The listing builds one solid part. Answer for the finished solid, in the listing's coordinates (mm). A direction names the side the tool comes from. Give positions to 0.01 mm unless a question says otherwise; leave off trailing zeros. Order: outer loops, then holes, each group sorted by start corner. A loop starts at its lowest first (then second) coordinate and runs counter-clockwise, first axis right, second up. Notation, with made-up numbers: (-31, -22) - (12, -22) arc R8 ccw to (12, -17) - close; hole circle Ø11 at (80, -27). An arc over 180 degrees is marked (long way). Answer as a JSON object with one key per item and string values. Group by question number.
Q1. Given pin 1 (12 mm diameter, centred on x = -0.5, y = 24.5, fed in from +Z); pin 2 (1 mm diameter, centred on x = 4.5, z = 24, fed in from +Y); pin 3 (4.5 mm diameter, centred on y = 32.5, z = 0, fed in from -X), each flat-ended and moving along its own axis, determine where each tip first touches the part or whether it passes through.
Q2. The mould has two halves that part along X. Classify faces 1 (the face through (-24, 0, 0)), 2 (the face through (0.215, 34.136, -18.768)), 3 (the face through (-20, 31, -1)): released by +X, released by -X, zero draft, split by the parting line, or undercut.
Q3. A cutting plane is placed at B-B, the plane y = 3. Give the vertices of the cut face in (x, z).
Q4. Consider line 1 (X direction, y = 34, z = 7); line 2 (X direction, y = 3.5, z = 17); line 3 (Z direction, x = 8, y = 8). Determine where each line is inside the solid, lowest interval first.
Q5. A cutting plane is placed at A-A, the plane z = 0. Count the separate pieces of the cut face and the enclosed holes in it, and give its area (3 significant figures).
Q6. For faces 4 (the face through (22.5, 9, 0)), 5 (the face through (0, 0, -24)), 6 (the face through (-0.2, 34.3, 17.5)), 7 (the face through (0, 18, 23)), determine the directions among +Z, -Z, +X, -X, +Y, -Y from which every point of the face is accessible in a straight line to the end or side of a thin tool.
Autodesk Inventor part; units mm, degrees
ref_plane "Work Plane1" through (0, 17.75, 0) normal (0, 1, 0) x (1, 0, 0)
ref_plane "YZ Plane" through (0, 0, 0) normal (1, 0, 0) x (0, 1, 0)
ref_plane "XZ Plane" through (0, 0, 0) normal (0, 1, 0) x (-1, 0, 0)
sketch "Sketch1" plane through (0, 0, 0) normal (0, 1, 0) x (-1, 0, 0)
  line L0 (25, 25) -> (-25, 25)
  line L1 (-25, 25) -> (-25, -25)
  line L2 (-25, -25) -> (25, -25)
  line L3 (25, -25) -> (25, 25)
  line L4 (25, 25) -> (-25, -25) construction
  line L5 (-25, 25) -> (25, -25) construction
  line L6 (-22.5, 22.5) -> (22.5, 22.5)
  line L7 (22.5, 22.5) -> (22.5, -22.5)
  line L8 (22.5, -22.5) -> (-22.5, -22.5)
  line L9 (-22.5, -22.5) -> (-22.5, 22.5)
  line L10 (-22.5, 22.5) -> (22.5, -22.5) construction
  line L11 (22.5, 22.5) -> (-22.5, -22.5) construction
  point P0 (0, 0)
  dimension "d0" = 50
  dimension "d1" = 50
  dimension "d2" = 45
  dimension "d3" = 45
extrude "Extrusion1" add sketch "Sketch1" along normal blind 30
extrude "Extrusion2" add sketch "Sketch1" along normal blind 2 contours L6 L7 L8 L9
sketch "Sketch2" plane through (0, 30, 0) normal (0, 1, 0) x (1, 0, 0)
  point P0 (0, 0)
sketch "Sketch3" plane through (0, 30, 0) normal (0, 1, 0) x (1, 0, 0)
  line L0 (17.5, -17.5) -> (-17.5, -17.5)
  line L1 (-17.5, -17.5) -> (-17.5, 17.5)
  line L2 (-17.5, 17.5) -> (17.5, 17.5)
  line L3 (17.5, 17.5) -> (17.5, -17.5)
  line L4 (17.5, -17.5) -> (-17.5, 17.5) construction
  line L5 (-17.5, -17.5) -> (17.5, 17.5) construction
  line L6 (-25, 25) -> (-25, -25)
  line L7 (25, -25) -> (-25, -25)
  line L8 (-25, -25) -> (-25, 25)
  line L9 (-25, 25) -> (25, 25)
  line L10 (25, 25) -> (25, -25)
  line L11 (25, -25) -> (-25, 25) construction
  line L12 (-25, -25) -> (25, 25) construction
  point P0 (0, 0)
  dimension "d8" = 35
  dimension "d9" = 35
extrude "Extrusion3" add sketch "Sketch3" along normal blind 5.5
ref_plane "Work Plane1" through (0, 17.75, 0) normal (0, 1, 0) x (1, 0, 0)
chamfer "Chamfer1" distance 5 distance2 13.25 4 edges at (22.5, 30, 0) (0, 30, -22.5) (-22.5, 30, 0) (0, 30, 22.5) measured on face at (-5.8333, 30, 20.8333)
sketch "Sketch5" plane through (0, 35.5, 0) normal (0, 1, 0) x (1, 0, 0)
  point P0 (0, 0)
sketch "Sketch6" plane through (-17.5, 35.5, -17.5) normal (0, 0, 1) x (1, 0, 0)
  circle A0 centre (17.5, -3) radius 1.5
  line L0 (0, 0) -> (35, 0)
  point P0 (17.5, -35.5)
  point P1 (17.5, 0)
  dimension "d21" = 3
  dimension "d30" = 3
extrude "Extrusion5" cut sketch "Sketch6" against normal through all
sketch "Sketch7" plane through (0, 35.5, 0) normal (0, 1, 0) x (1, 0, 0)
  line L0 (25, 25) -> (-25, 25)
  line L1 (10, 25) -> (0, 25)
  line L2 (10, 25) -> (-10, 25)
  line L3 (-10, 25) -> (10, 25)
  line L4 (10, 25) -> (10, 23)
  line L5 (10, 23) -> (-10, 23)
  line L6 (-10, 23) -> (-10, 25)
  point P0 (0, 0)
  dimension "d24" = 20
  dimension "d25" = 2
extrude "Extrusion6" cut sketch "Sketch7" against normal through all
sketch "Sketch9" plane through (10, 35.5, -23) normal (0, 0, -1) x (-1, 0, 0)
  circle A0 centre (10, -3) radius 1.5
  circle A1 centre (10, -3) radius 2.5
  point P0 (10, -35.5)
  dimension "d37" = 3
extrude "Extrusion7" cut sketch "Sketch9" against normal blind 3
pattern_circular "Circular Pattern2" count 4 over 360 about axis through (0, -10, 0) along (0, 1, 0) of "Extrusion7", "Extrusion6", "Extrusion5"
sketch "Sketch11" plane through (0, 32.5, -20) normal (0, 0, -1) x (-1, 0, 0)
  circle A0 centre (0, 0) radius 1.65
  circle A1 centre (0, 0) radius 2.65
  point P0 (0, -32.5)
  dimension "d38" = 3.3
  dimension "d39" = 5.3
extrude "Extrusion9" cut sketch "Sketch11" against normal through all contours A0
extrude "Extrusion10" cut sketch "Sketch11" along normal blind 4
sketch "Sketch12" plane through (0, 32.5, 20) normal (0, 0, 1) x (1, 0, 0)
  circle A0 centre (0, 0) radius 2.65
  point P0 (0, -32.5)
  dimension "d44" = 5.3
extrude "Extrusion11" cut sketch "Sketch12" along normal blind 9
sketch "Sketch13" plane through (-20, 32.5, 0) normal (-1, 0, 0) x (0, 0, 1)
  circle A0 centre (0, 0) radius 1.65
  circle A1 centre (0, 0) radius 2.65
  point P0 (0, -32.5)
  dimension "d47" = 3.3
  dimension "d48" = 5.3
extrude "Extrusion12" cut sketch "Sketch13" against normal through all contours A0
extrude "Extrusion13" cut sketch "Sketch13" along normal blind 9 contours A0 | A1
sketch "Sketch14" plane through (20, 32.5, 0) normal (1, 0, 0) x (0, 0, -1)
  circle A0 centre (0, 0) radius 2.65
  point P0 (0, -32.5)
  dimension "d53" = 5.3
extrude "Extrusion14" cut sketch "Sketch14" along normal blind 8.5
sketch "Sketch15" plane through (0, 35.5, 0) normal (0, 1, 0) x (1, 0, 0)
  line L0 (17.5, 17.5) -> (17.5, -17.5)
  line L1 (17.5, -17.5) -> (17.5, 17.5)
  line L2 (17.5, 17.5) -> (-17.5, 17.5)
  line L3 (-17.5, 17.5) -> (-17.5, -17.5)
  line L4 (-17.5, -17.5) -> (17.5, -17.5)
  line L5 (10, -23) -> (-10, -23)
  line L6 (10, -23) -> (10, -25)
  line L7 (10, -25) -> (25, -25)
  line L8 (25, -25) -> (25, -10)
  line L9 (23, -10) -> (23, 10)
  line L10 (25, -10) -> (23, -10)
  line L11 (23, -10) -> (23, 10)
  line L12 (23, 10) -> (25, 10)
  line L13 (25, 25) -> (10, 25)
  line L14 (25, 10) -> (25, 25)
  line L15 (25, 25) -> (10, 25)
  line L16 (10, 23) -> (-10, 23)
  line L17 (10, 25) -> (10, 23)
  line L18 (10, 23) -> (-10, 23)
  line L19 (-10, 23) -> (-10, 25)
  line L20 (-10, 25) -> (-25, 25)
  line L21 (-10, 25) -> (-25, 25)
  line L22 (-25, 25) -> (-25, 10)
  line L23 (-23, 10) -> (-23, -10)
  line L24 (-25, 10) -> (-23, 10)
  line L25 (-23, 10) -> (-23, -10)
  line L26 (-23, -10) -> (-25, -10)
  line L27 (-25, -10) -> (-25, -25)
  line L28 (-10, -23) -> (10, -23)
  line L29 (-10, -25) -> (-10, -23)
  line L30 (-10, -23) -> (-10, -25)
  line L31 (-10, -25) -> (-25, -25)
  point P0 (0, 0)
  dimension "d56" = 15
  dimension "d57" = 15
extrude "Extrusion15" add sketch "Sketch15" along normal blind 0.5
extrude "Extrusion16" add sketch "Sketch1" against normal blind 2 contours L3 L2 L1 L0 | L6 L7 L8 L9
sketch "Sketch16" plane through (0, -2, 0) normal (0, -1, 0) x (1, 0, 0)
  line L0 (-15.5086, 20.4473) -> (19.4914, 20.4473) construction
  line L1 (19.4914, 20.4473) -> (19.4914, -17.6327) construction
  line L2 (19.4914, -17.6327) -> (-15.5086, -17.6327) construction
  line L3 (-15.5086, -17.6327) -> (-15.5086, 20.4473) construction
  point P0 (0, 0)
  dimension "d73" = 35
properties part number "Ulepszona wersja"
Reply:
{
 "1": {"pin 1": "stops at z = 23", "pin 2": "stops at y = 0", "pin 3": "stops at x = -20"},
 "2": {"face 1": "zero draft", "face 2": "undercut", "face 3": "released by -X"},
 "3": {"outline": "(-25, -25) - (-10, -25) - (-10, -23) - (10, -23) - (10, -25) - (25, -25) - (25, -10) - (23, -10) - (23, 10) - (25, 10) - (25, 25) - (10, 25) - (10, 23) - (-10, 23) - (-10, 25) - (-25, 25) - (-25, 10) - (-23, 10) - (-23, -10) - (-25, -10) - close; hole (-22.5, -22.5) - (22.5, -22.5) - (22.5, 22.5) - (-22.5, 22.5) - close"},
 "4": {"line 1": "x = -23 to -17.5, 17.5 to 23", "line 2": "x = -25 to -22.5, 22.5 to 25", "line 3": "z = -23 to -22.5, 22.5 to 23"},
 "5": {"separate pieces": "3", "enclosed holes": "0", "area": "304 mm^2"},
 "6": {"face 4": "none", "face 5": "-Z, +Y", "face 6": "+Y", "face 7": "+Z, +Y"}
}
